Can you work these out from the drawing? Everything is in mm from the part's minimum corner. Give positions to 0.01 mm unless a question says otherwise; leave off trailing zeros. Loops run counter-clockwise (first coordinate to the right, second up) from the corner with the lowest first, then second, coordinate; pieces in that order, holes last.
Q1. I need wall thicknesses on line 1 (Z direction, x = 0.1, y = 2.9); line 2 (Y direction, x = 0.8, z = 7.5). Which ranges of each line are inside material? Lowest first, please.
Q2. If we section it at B-B (y = 2.65): Please give me the cut outline in (x, z).
Q3. If we section it at A-A (x = 0.55): Please give me the cut outline in (y, z).
Q4. We'd pull the mould along Y, two halves only. Please class the marked faces 1, 2, 3 and 4: +Y half, -Y half, draft (parallel to the pull), parting line (faces both ways), or undercut.
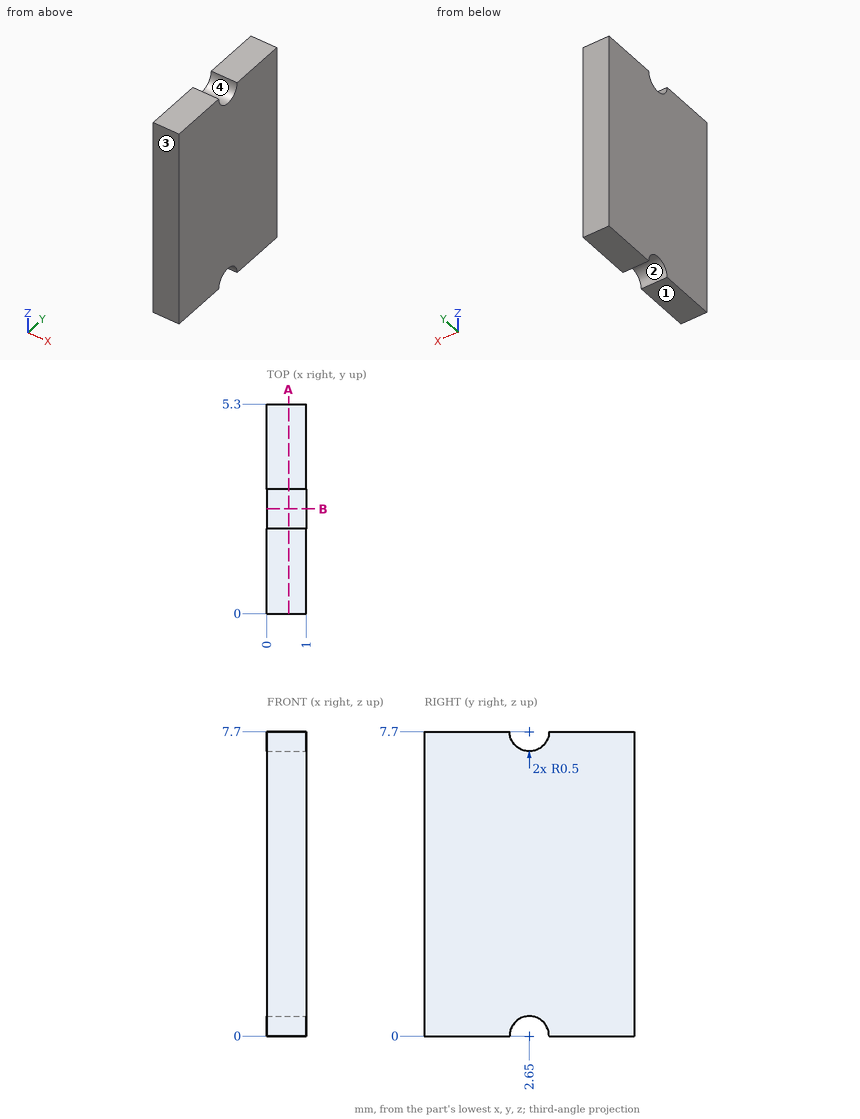
Check sheet entries:
1. line 1: z = 0.43 to 7.27
1. line 2: y = 0 to 2.19, 3.11 to 5.3
2. outline: (0, 0.5) - (1, 0.5) - (1, 7.2) - (0, 7.2) - close
3. outline: (0, 0) - (2.15, 0) arc R0.5 cw to (3.15, 0) - (5.3, 0) - (5.3, 7.7) - (3.15, 7.7) arc R0.5 cw to (2.15, 7.7) - (0, 7.7) - close
4. face 1: draft
4. face 2: undercut
4. face 3: -Y half
4. face 4: undercut
